from build123d import *

# Parameters (mm, degrees)
SKETCH2_R      = 3.175
EXTRUDE1_DEPTH = 38.1
SKETCH3_W      = 57.15
SKETCH3_H      = 11.176
EXTRUDE2_DEPTH = 33.4645
SKETCH4_W      = 57.15
SKETCH4_H      = 16.764
EXTRUDE3_DEPTH = 29.6545
SKETCH5_R      = 4.7625
EXTRUDE4_DEPTH = 26.4
EXTRUDE5_DEPTH = 26.4


with BuildPart() as part:
    # Sketch2 → Extrude1 (new body)
    with BuildSketch(Plane.XY):
        Polygon((-22.225, 12.7), (-28.575, 12.7), (-28.575, -12.7), (-22.225, -12.7), (22.225, -12.7), (28.575, -12.7), (28.575, 12.7), (22.225, 12.7), align=None)
        with Locations((19.05, 0)):
            Circle(SKETCH2_R, mode=Mode.SUBTRACT)
        with Locations((-19.05, 0)):
            Circle(SKETCH2_R, mode=Mode.SUBTRACT)
    extrude(amount=EXTRUDE1_DEPTH)

    # Sketch3 → Extrude2 (cut)
    with BuildSketch(Plane.XY.offset(38.1)):
        Rectangle(SKETCH3_W, SKETCH3_H)
    extrude(amount=-EXTRUDE2_DEPTH, mode=Mode.SUBTRACT)

    # Sketch4 → Extrude3 (cut)
    with BuildSketch(Plane.XY.offset(38.1)):
        Rectangle(SKETCH4_W, SKETCH4_H)
    extrude(amount=-EXTRUDE3_DEPTH, mode=Mode.SUBTRACT)

    # Sketch5 → Extrude4 (cut, through all)
    with BuildSketch(Plane(origin=(0, 12.7, 0), x_dir=(-1, 0, 0), z_dir=(0, 1, 0))):
        with Locations((0, 22.225)):
            Circle(SKETCH5_R)
    extrude(amount=-EXTRUDE4_DEPTH, mode=Mode.SUBTRACT)

    # Sketch6 → Extrude5 (cut, through all)
    with BuildSketch(Plane(origin=(0, 12.7, 0), x_dir=(1, 0, 0), z_dir=(0, 1, 0))):
        with BuildLine():
            Line((-28.575, -9.525), (-28.575, -38.1))
            Line((-28.575, -38.1), (28.575, -38.1))
            Line((28.575, -38.1), (28.575, -9.525))
            ThreePointArc((28.575, -9.525), (22.913958086, -13.508463236), (19.05, -19.25173781))
            ThreePointArc((19.05, -19.25173781), (0, -31.75), (-19.05, -19.25173781))
            ThreePointArc((-19.05, -19.25173781), (-22.913958086, -13.508463236), (-28.575, -9.525))
        make_face()
    extrude(amount=-EXTRUDE5_DEPTH, mode=Mode.SUBTRACT)


solid = part.part
Read the model definition and answer for the solid it produces. Units are mm, in the model's axes. A direction names the side the tool comes from. Coordinates: 2 decimals unless noted, no trailing zeros. Write each loop counter-clockwise with the first axis right and the second up, starting at its lowest first coordinate (ties: lowest second). Pieces come first, ordered by that corner, then holes. Notation, with made-up numbers: (23.25, 19) - (39.25, 19) arc R17 ccw to (39.25, 44) - close; hole circle Ø10 at (-36.75, 0.25). An arc over 180 degrees is marked (long way). One line per question, with ' | ' between items.
Q1. Determine the mould class of faces 3 (the cylindrical face through (-16.02, 0.95, 2.29)), 4 (the cylindrical face through (0.62, 10.571, 26.947)), 5 (the flat face through (0, 0, 4.636)) for opening direction Z: +Z half, -Z half, draft (parallel to the pull), parting line (faces both ways), or undercut.
Result set:
face 3: draft | face 4: undercut | face 5: +Z half
Q2. Find section B-B, the plane z = 5.5. Write down the section's boundary in (x, y) (3 decimals).
Result set:
outline: (-28.575, -12.7) - (28.575, -12.7) - (28.575, -5.588) - (-28.575, -5.588) - close; (-28.575, 5.588) - (28.575, 5.588) - (28.575, 12.7) - (-28.575, 12.7) - close
Q3. Each of these flat-tipped pins is pushed along its axis until it touches: P1, Ø2, axis at x = -5, y = -7, coming from the +Z side; P2, Ø10, axis at y = -1.5, z = 19, coming from the -X side; P3, Ø4, axis at y = -9.5, z = 14.5, coming from the +X side. Where does it stop, or does it pass through?
Result set:
P1: z = 8.45 | P2: through | P3: x = 23.98
Q4. Find section D-D, the plane x = -16.5. Write down the section's boundary in (y, z).
Result set:
outline: (-12.7, 0) - (-1.89, 0) - (-1.89, 4.64) - (-5.59, 4.64) - (-5.59, 8.45) - (-8.38, 8.45) - (-8.38, 23.59) - (-12.7, 23.59) - close; (1.89, 0) - (12.7, 0) - (12.7, 23.59) - (8.38, 23.59) - (8.38, 8.45) - (5.59, 8.45) - (5.59, 4.64) - (1.89, 4.64) - close
Q5. Find section A-A, the plane x = 0. Write down the section's boundary in (y, z), plus the area to 3 significant figures.
Result set:
outline: (-12.7, 0) - (12.7, 0) - (12.7, 17.46) - (8.38, 17.46) - (8.38, 8.45) - (5.59, 8.45) - (5.59, 4.64) - (-5.59, 4.64) - (-5.59, 8.45) - (-8.38, 8.45) - (-8.38, 17.46) - (-12.7, 17.46) - close; (-12.7, 26.99) - (-8.38, 26.99) - (-8.38, 31.75) - (-12.7, 31.75) - close; (8.38, 26.99) - (12.7, 26.99) - (12.7, 31.75) - (8.38, 31.75) - close | area: 291 mm^2
Q6. For faces 1 (the cylindrical face through (0.62, -10.511, 26.947)), 2 (the flat face through (0, -5.588, 7)), determine the directions among +Z, -Z, +X, -X, +Y, -Y from which every point of the face is accessible in a straight line to the end or side of a thin tool.
Result set:
face 1: +Y, -Y | face 2: +Z, +X, -X
Q7. Consider L1, parallel to X at y = -0.25, z = 4 (3 decimals); L2, parallel to Y at x = 26, z = 5.5; L3, parallel to Y at x = -9, z = 10.5. Determine where each line is inside the solid, lowest interval first. Write a range as [from, to].
Result set:
L1: [-28.575, -22.215], [-15.885, 15.885], [22.215, 28.575] | L2: [-12.7, -5.59], [5.59, 12.7] | L3: [-12.7, -8.38], [8.38, 12.7]
